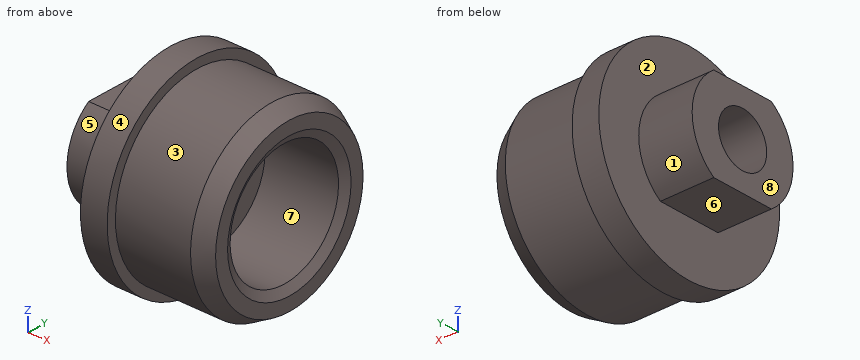
```python
from build123d import *

# Parameters (mm, degrees)
SKETCH1_R           = 6.9215
BOSS_EXTRUDE1_DEPTH = 6.985
SKETCH2_R           = 7.62
BOSS_EXTRUDE2_DEPTH = 2.032
SKETCH3_R           = 4.2545
BOSS_EXTRUDE3_DEPTH = 4.064
CUT_EXTRUDE1_START  = -4.064
CUT_EXTRUDE1_DEPTH  = 4.064
SKETCH5_R           = 2.032
CUT_EXTRUDE2_DEPTH  = 17.948196394
SKETCH6_R           = 4.572
CUT_EXTRUDE3_DEPTH  = 5.969
CHAMFER1_SIZE       = 1.27
CHAMFER1_SIZE2      = 0.703972495
CHAMFER2_SIZE       = 0.635
CHAMFER2_SIZE2      = 0.381546493


with BuildPart() as part:
    # Sketch1 → Boss-Extrude1 (new body)
    with BuildSketch(Plane(origin=(0, 0, 0), x_dir=(0, 0, -1), z_dir=(1, 0, 0))):
        Circle(SKETCH1_R)
    extrude(amount=-BOSS_EXTRUDE1_DEPTH)

    # Sketch2 → Boss-Extrude2 (add)
    with BuildSketch(Plane.ZY.offset(6.985)):
        Circle(SKETCH2_R)
    extrude(amount=BOSS_EXTRUDE2_DEPTH)

    # Sketch3 → Boss-Extrude3 (add)
    with BuildSketch(Plane.ZY.offset(9.017)):
        Circle(SKETCH3_R)
    extrude(amount=BOSS_EXTRUDE3_DEPTH)

    # Sketch4 → Cut-Extrude1 (cut)
    with BuildSketch(Plane.ZY.offset(13.081).offset(CUT_EXTRUDE1_START)):
        with BuildLine():
            Line((-3.4925, -2.429653062), (-3.4925, 2.429653062))
            ThreePointArc((-3.4925, 2.429653062), (-4.2545, 0), (-3.4925, -2.429653062))
        make_face()
        with BuildLine():
            ThreePointArc((4.2545, 0), (4.059532701, 1.273171041), (3.4925, 2.429653062))
            Line((3.4925, 2.429653062), (3.4925, -2.429653062))
            ThreePointArc((3.4925, -2.429653062), (4.059532701, -1.273171041), (4.2545, 0))
        make_face()
    extrude(amount=CUT_EXTRUDE1_DEPTH, mode=Mode.SUBTRACT)

    # Sketch5 → Cut-Extrude2 (cut, through all)
    with BuildSketch(Plane.ZY.offset(13.081)):
        Circle(SKETCH5_R)
    extrude(amount=-CUT_EXTRUDE2_DEPTH, mode=Mode.SUBTRACT)

    # Sketch6 → Cut-Extrude3 (cut)
    with BuildSketch(Plane(origin=(0, 0, 0), x_dir=(0, 0, -1), z_dir=(1, 0, 0))):
        Circle(SKETCH6_R)
    extrude(amount=-CUT_EXTRUDE3_DEPTH, mode=Mode.SUBTRACT)

    # Chamfer1
    chamfer1_edges = [part.edges().sort_by_distance(p)[0] for p in [
        (0, 0, 6.9215),
    ]]
    chamfer1_side = [part.faces().sort_by_distance(p)[0] for p in [
        (-3.4925, 0, 6.9215),
    ]]
    chamfer(chamfer1_edges, length=CHAMFER1_SIZE, length2=CHAMFER1_SIZE2, reference=chamfer1_side[0])

    # Chamfer2
    chamfer2_edges = [part.edges().sort_by_distance(p)[0] for p in [
        (0, 0, 4.572),
    ]]
    chamfer2_side = [part.faces().sort_by_distance(p)[0] for p in [
        (0, 0, 6.04166927),
    ]]
    chamfer(chamfer2_edges, length=CHAMFER2_SIZE, length2=CHAMFER2_SIZE2, reference=chamfer2_side[0])


solid = part.part
```
Input: part model. Units: mm. Frame: model coordinates. Face numbers are marked on the shaded views. A direction names the side the tool comes from. Round coordinates to 2 decimals unless told otherwise and drop trailing zeros. Order: outer loops, then holes, each group sorted by start corner. A loop starts at its lowest first (then second) coordinate and runs counter-clockwise, first axis right, second up. Notation, with made-up numbers: (44, 10.25) - (96, 10.25) arc R23 ccw to (96, 34.25) - close; hole circle Ø8 at (79.5, -0.75). An arc over 180 degrees is marked (long way). One line per question, with ' | ' between items. Start each with the question number.
1) Set-up query: the marked faces 1, 2, 3, 4 and 5. Return all of +Z, -Z, +X, -X, +Y, -Y with unobstructed straight access to the full face (end or side cutting, diameter ignored); none if empty.
2) Ray query, probe 1 along Y at (x, z) = (-8.25, 0); probe 2 along Y at (x, z) = (-1.85, 0); probe 3 along X at (y, z) = (-5.5, 4.5) (3 decimals). Return the intervals inside material, ascending.
3) Pull-direction query (Z, two-part tool) for the marked faces 6, 7 and 8; classes: +Z half, -Z half, draft (parallel to the pull), parting line (faces both ways), or undercut.
4) Cut plane A-A, the plane z = 0. Return the cut outline in (x, y) (1 decimal).
5) Contact query for flat-ended pins moving along their axis: P1, Ø6, axis at x = -6.5, z = -0.5, coming from the -Y side; P2, Ø5, axis at x = -9, y = 3.5, coming from the +Z side; P3, Ø4.5, axis at y = -2, z = -1.5, coming from the +X side; P4, Ø1, axis at x = -11, y = -4, coming from the -Z side. Output: stop coordinate, or through.
6) Cut plane D-D, the plane x = -6.5. Return the cut outline in (y, z), then the cut area to 3 significant figures.
7) Cut plane C-C, the plane x = -9.75. Return the cut outline in (y, z).
8) Cut plane B-B, the plane y = 0. Return the cut outline in (x, z) (1 decimal).
Worked out:
1) face 1: -X, +Y | face 2: -X | face 3: +X | face 4: +X, -X | face 5: -X, -Y
2) probe 1: y = -7.62 to -2.03, 2.03 to 7.62 | probe 2: y = -6.92 to -4.57, 4.57 to 6.92 | probe 3: x = -9.017 to -6.985
3) face 6: -Z half | face 7: undercut | face 8: draft
4) outline: (-13.1, -4.3) - (-9, -4.3) - (-9, -7.6) - (-7, -7.6) - (-7, -6.9) - (-1.3, -6.9) - (0, -6.2) - (0, -5.2) - (-0.4, -4.6) - (-6, -4.6) - (-6, -2) - (-13.1, -2) - close; (-13.1, 2) - (-6, 2) - (-6, 4.6) - (-0.4, 4.6) - (0, 5.2) - (0, 6.2) - (-1.3, 6.9) - (-7, 6.9) - (-7, 7.6) - (-9, 7.6) - (-9, 4.3) - (-13.1, 4.3) - close
5) P1: stops at y = -7.62 | P2: stops at z = 7.55 | P3: stops at x = -0.27 | P4: stops at z = -2.42
6) outline: circle Ø13.84 at (0, 0); hole circle Ø4.06 at (0, 0) | area: 138 mm^2
7) outline: (-2.43, -3.49) - (2.43, -3.49) arc R4.25 ccw to (2.43, 3.49) - (-2.43, 3.49) arc R4.25 ccw to start; hole circle Ø4.06 at (0, 0)
8) outline: (-13.1, -3.5) - (-9, -3.5) - (-9, -7.6) - (-7, -7.6) - (-7, -6.9) - (-1.3, -6.9) - (0, -6.2) - (0, -5.2) - (-0.4, -4.6) - (-6, -4.6) - (-6, -2) - (-13.1, -2) - close; (-13.1, 2) - (-6, 2) - (-6, 4.6) - (-0.4, 4.6) - (0, 5.2) - (0, 6.2) - (-1.3, 6.9) - (-7, 6.9) - (-7, 7.6) - (-9, 7.6) - (-9, 3.5) - (-13.1, 3.5) - close
